from build123d import *
from build123d.topology import SkipClean

# Parameters (mm, degrees)
BOSS_EXTRUDE1_DEPTH = 40
BOSS_EXTRUDE2_START = 5
BOSS_EXTRUDE2_DEPTH = 5
SKETCH4_R           = 5
SKETCH4_R_2         = 2.5
BOSS_EXTRUDE3_DEPTH = 40
CUT_EXTRUDE2_START  = -60
SKETCH5_R           = 2.5
SKETCH5_R_2         = 2.456644978
CUT_EXTRUDE2_DEPTH  = 60


with BuildPart() as part:
    # Sketch1 → Boss-Extrude1 (new body)
    with BuildSketch(Plane.XY):
        with BuildLine():
            Line((-95, -45), (-95, 45))
            ThreePointArc((-95, 45), (-92.071067812, 52.071067812), (-85, 55))
            Line((-85, 55), (85, 55))
            ThreePointArc((85, 55), (92.071067812, 52.071067812), (95, 45))
            Line((95, 45), (95, -45))
            ThreePointArc((95, -45), (92.071067812, -52.071067812), (85, -55))
            Line((85, -55), (-85, -55))
            ThreePointArc((-85, -55), (-92.071067812, -52.071067812), (-95, -45))
        make_face()
        with BuildLine():
            Line((-85, -50), (85, -50))
            ThreePointArc((85, -50), (88.535533906, -48.535533906), (90, -45))
            Line((90, -45), (90, 45))
            ThreePointArc((90, 45), (88.535533906, 48.535533906), (85, 50))
            Line((85, 50), (-85, 50))
            ThreePointArc((-85, 50), (-88.535533906, 48.535533906), (-90, 45))
            Line((-90, 45), (-90, -45))
            ThreePointArc((-90, -45), (-88.535533906, -48.535533906), (-85, -50))
        make_face(mode=Mode.SUBTRACT)
    extrude(amount=BOSS_EXTRUDE1_DEPTH)

    # Sketch3 → Boss-Extrude2 (add)
    with BuildSketch(Plane(origin=(0, 0, 0), x_dir=(-1, 0, 0), z_dir=(0, 0, -1)).offset(BOSS_EXTRUDE2_START)):
        with BuildLine():
            Line((-85, -55), (85.025805787, -55))
            ThreePointArc((85.025805787, -55), (92.096873598, -52.071067812), (95.025805787, -45))
            Line((95.025805787, -45), (95.025805787, 45))
            ThreePointArc((95.025805787, 45), (92.096873598, 52.071067812), (85.025805787, 55))
            Line((85.025805787, 55), (-85, 55))
            ThreePointArc((-85, 55), (-92.071067812, 52.071067812), (-95, 45))
            Line((-95, 45), (-95, -45))
            ThreePointArc((-95, -45), (-92.071067812, -52.071067812), (-85, -55))
        make_face()
    extrude(amount=-BOSS_EXTRUDE2_DEPTH)

    # Sketch4 → Boss-Extrude3 (add)
    # profile 1 of 4: a face of its own
    with BuildSketch(Plane.XY):
        with Locations(Location((-79.484929462, 40.691862401, 0), (0, 0, 180))):
            Circle(SKETCH4_R)
        with Locations((-79.484929462, 40.691862401)):
            Circle(SKETCH4_R_2, mode=Mode.SUBTRACT)
    # profile 2 of 4: a face of its own
    with BuildSketch(Plane.XY):
        with Locations(Location((-79.484929462, -41.238061896, 0), (0, 0, 180))):
            Circle(SKETCH4_R)
        with Locations((-79.484929462, -41.238061896)):
            Circle(SKETCH4_R_2, mode=Mode.SUBTRACT)
    # profile 3 of 4: a face of its own
    with BuildSketch(Plane.XY):
        with Locations(Location((79.186023927, -41.238061896, 0), (0, 0, 180))):
            Circle(SKETCH4_R)
        with Locations((79.186023927, -41.238061896)):
            Circle(SKETCH4_R_2, mode=Mode.SUBTRACT)
    # profile 4 of 4: a face of its own
    with BuildSketch(Plane.XY):
        with Locations(Location((79.186023927, 40.691862401, 0), (0, 0, 180))):
            Circle(SKETCH4_R)
        with Locations((79.186023927, 40.691862401)):
            Circle(SKETCH4_R_2, mode=Mode.SUBTRACT)
    extrude(amount=BOSS_EXTRUDE3_DEPTH)

    # Sketch5 → Cut-Extrude2 (cut)
    with SkipClean():  # the faces are left unmerged after this step: merging them gives an invalid solid
        with BuildSketch(Plane.XY.offset(40).offset(CUT_EXTRUDE2_START)):
            with Locations(Location((-79.484929462, 40.691862401, 0), (0, 0, 180))):
                Circle(SKETCH5_R)
            with Locations((79.186023927, 40.691862401)):
                Circle(SKETCH5_R_2)
            with Locations(Location((-79.484929462, -41.238061896, 0), (0, 0, 180))):
                Circle(SKETCH5_R)
            with Locations(Location((79.186023927, -41.238061896, 0), (0, 0, 180))):
                Circle(SKETCH5_R)
        extrude(amount=CUT_EXTRUDE2_DEPTH, mode=Mode.SUBTRACT)


solid = part.part
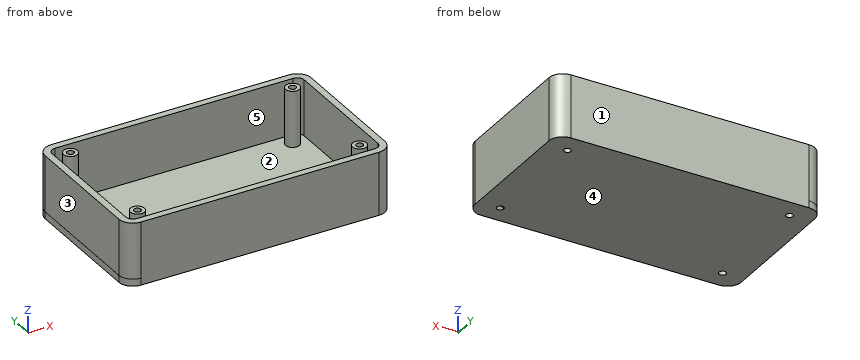
Geometry check sheet. Reference: the model listing, model coordinates, mm. Face numbers are marked on the shaded views. A direction names the side the tool comes from. Round coordinates to 2 decimals unless told otherwise and drop trailing zeros. Order: outer loops, then holes, each group sorted by start corner. A loop starts at its lowest first (then second) coordinate and runs counter-clockwise, first axis right, second up. Notation, with made-up numbers: M 59,-10 L 91,-10 A17 ccw 91,7 Z; hole C 61.25,-22.75 d10. An arc over 180 degrees is marked long. Answer in a Markdown table with one row per item. Add a question column.
Item 1: Set-up check for the marked faces 1 and 2: record each of +Z, -Z, +X, -X, +Y, -Y from which the full face is reachable in a straight line by a thin tool's end or side.
Item 2: Sectioned sample at C-C, the plane x = -55. Enter the section's corners in (y, z), plus the area to 3 significant figures.
Item 3: Material ranges on L1, parallel to X at y = 27, z = 32; L2, parallel to Y at x = -43, z = 8.5; L3, parallel to Y at x = -79.5, z = 3, recorded low to high. Write a range as [from, to].
Item 4: Depth check by flat-ended pin: pin 1 Ø1 at (y, z) = (26.5, 23.5) entering from -X. Enter the tip coordinate at first touch or a pass-through.
Item 5: Draft check along X on the marked faces 3, 4 and 5. Enter one of: released by +X, released by -X, zero draft, split by the parting line, or undercut.
Item 6: Sectioned sample at A-A, the plane z = 30. State how many separate pieces and enclosed holes the cut face has, plus the area to 3 significant figures.
Filled in:
| question | item | result |
|---|---|---|
| 1 | face 1 | +Z, -Z, +X, -X, +Y |
| 1 | face 2 | +Z |
| 2 | outline | M -55,-5 L 55,-5 L 55,40 L 50,40 L 50,0 L -50,0 L -50,40 L -55,40 Z |
| 2 | area | 950 mm² |
| 3 | L1 | x = [-95, -90], [90, 95] |
| 3 | L2 | y = [-55, -50], [50, 55] |
| 3 | L3 | y = [-55, -50], [-46.24, -43.74], [-38.74, -36.24], [35.69, 38.19], [43.19, 45.69], [50, 55] |
| 4 | pin 1 | stops at x = -95 |
| 5 | face 3 | released by -X |
| 5 | face 4 | zero draft |
| 5 | face 5 | undercut |
| 6 | separate pieces | 5 |
| 6 | enclosed holes | 5 |
| 6 | area | 3,070 mm² |
